Autodesk Inventor part; units mm, degrees
ref_plane "YZ Plane" through (0, 0, 0) normal (1, 0, 0) x (0, 1, 0)
ref_plane "XZ Plane" through (0, 0, 0) normal (0, 1, 0) x (-1, 0, 0)
ref_plane "XY Plane" through (0, 0, 0) normal (0, 0, 1) x (1, 0, 0)
sketch "Esquisse1" plane through (0, 0, 0) normal (0, 0, 1) x (1, 0, 0)
  line L0 (-368.5, -152.5) -> (368.5, -152.5)
  line L1 (368.5, -152.5) -> (368.5, 152.5)
  line L2 (368.5, 152.5) -> (-368.5, 152.5)
  line L3 (-368.5, 152.5) -> (-368.5, -152.5)
  line L4 (-368.5, -152.5) -> (368.5, 152.5) construction
  line L5 (-356, -140) -> (356, -140)
  line L6 (356, -140) -> (356, 140)
  line L7 (356, 140) -> (-356, 140)
  line L8 (-356, 140) -> (-356, -140)
  line L9 (-356, -140) -> (356, 140) construction
  circle A0 centre (-353.5, 137.5) radius 2.5
  circle A1 centre (-353.5, -137.5) radius 2.5
  circle A2 centre (353.5, -137.5) radius 2.5
  circle A3 centre (353.5, 137.5) radius 2.5
  line L10 (121.5, -10.5) -> (173.5, -10.5)
  line L11 (193.5, -30.5) -> (193.5, -82.5)
  line L12 (173.5, -102.5) -> (121.5, -102.5)
  line L13 (101.5, -82.5) -> (101.5, -30.5)
  line L14 (101.5, -10.5) -> (193.5, -102.5) construction
  line L15 (193.5, -10.5) -> (101.5, -102.5) construction
  line L16 (121.5, -10.5) -> (101.5, -30.5)
  line L17 (101.5, -82.5) -> (121.5, -102.5)
  line L18 (173.5, -102.5) -> (193.5, -82.5)
  line L19 (193.5, -30.5) -> (173.5, -10.5)
  circle A4 centre (106.25, -15.25) radius 2.2
  circle A5 centre (188.75, -15.25) radius 2.2
  circle A6 centre (188.75, -97.75) radius 2.2
  circle A7 centre (106.25, -97.75) radius 2.2
  point P0 (0, 0)
  point P1 (-356, -137.5)
  point P2 (-353.5, -140)
  point P3 (353.5, -140)
  point P4 (356, -137.5)
  point P5 (356, 137.5)
  point P6 (353.5, 140)
  point P7 (-356, 137.5)
  point P8 (-353.5, 140)
  point P9 (147.5, -56.5)
  dimension "d0" = 737
  dimension "d1" = 305
  dimension "d2" = 12.5
  dimension "d3" = 12.5
  dimension "d4" = 5
  dimension "d7" = 5
  dimension "d8" = 5
  dimension "d9" = 5
  dimension "d36" = 92
  dimension "d37" = 92
  dimension "d38" = 50
  dimension "d39" = 175
  dimension "d48" = 20
  dimension "d49" = 20
  dimension "d50" = 20
  dimension "d51" = 20
  dimension "d52" = 20
  dimension "d53" = 20
  dimension "d54" = 20
  dimension "d55" = 20
  dimension "d57" = 4.4
  dimension "d58" = 4.4
  dimension "d59" = 4.4
  dimension "d60" = 4.4
  dimension "d61" = 4.75
  dimension "d62" = 4.75
extrude "Extrusion1" add sketch "Esquisse1" along normal blind 2 contours L3 L2 L1 L0 | L8 A1 L5 | A1 L8 A0 L7 A3 L6 A2 L5 | A2 L6 L5 | L8 L7 A0 | A3 L7 L6
properties part number "PlaqueVentilo"
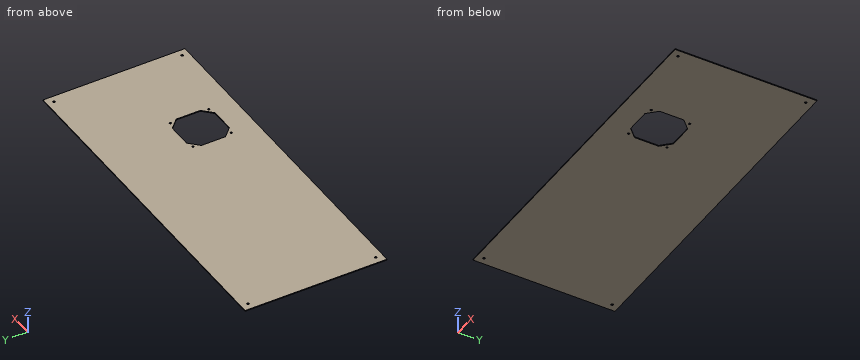
Design review of the part built by this model. Coordinates are the model's own, in mm. Round coordinates to 2 decimals unless told otherwise and drop trailing zeros. Write each loop counter-clockwise with the first axis right and the second up, starting at its lowest first coordinate (ties: lowest second). Pieces come first, ordered by that corner, then holes.
Item 1: Consider section B-B on z = 0.45. Count the separate pieces of the cut face and the enclosed holes in it, and give its area (3 significant figures).
Item 2: For pin 1 Ø4 at (x, y) = (-353.5, 137.5) entering from +Z, flat-tipped, find the tip position at first contact; note if it passes through.
Item 3: Wall thickness on L1, parallel to X at y = 137.5, z = 1.3; L2, parallel to Y at x = 106.25, z = 0.4; L3, parallel to Y at x = 353.5, z = 0.55: over which ranges is each line inside the solid? List them lowest first.
Item 4: Consider section A-A on x = 138. Give the boundary of the cut face in (y, z).
Check values:
1. separate pieces: 1
1. enclosed holes: 9
1. area: 217,000 mm2
2. pin 1: passes through
3. L1: x = -368.5 to -356, -351 to 351, 356 to 368.5
3. L2: y = -152.5 to -99.95, -95.55 to -87.25, -25.75 to -17.45, -13.05 to 152.5
3. L3: y = -152.5 to -140, -135 to 135, 140 to 152.5
4. outline: (-152.5, 0) - (-102.5, 0) - (-102.5, 2) - (-152.5, 2) - close; (-10.5, 0) - (152.5, 0) - (152.5, 2) - (-10.5, 2) - close
